```python
from build123d import *

# Parameters (mm, degrees)
SKETCH_1_W             = 230.160423268
SKETCH_1_H             = 76.880643476
SM_BASE_FLANGE_1_DEPTH = 1
OTHER_START            = -38.440321738
OTHER_1_DEPTH          = 76.880643476
OTHER_1_2_DEPTH        = 76.880643476


# Read off the part's stored shape, not the designer's step: 转折1
# Sheet-metal steps are written as plain solids
with BuildPart() as part:
    # Sketch 1 → 基体-法兰1 (new body)
    with BuildSketch(Plane(origin=(0, 0, 0), x_dir=(1, 0, 0), z_dir=(0, 1, 0))):
        Rectangle(SKETCH_1_W, SKETCH_1_H)
    extrude(amount=-SM_BASE_FLANGE_1_DEPTH)

    # Other 1 outline → Other 1 (cut)
    with BuildSketch(Plane.XY.offset(OTHER_START)):
        with BuildLine():
            Line((115.080211634, 0), (0.093295252, 0))
            ThreePointArc((0.093295252, 0), (-1.033318835, -0.740370349), (-2.35619449, -1))
            Line((-2.35619449, -1), (115.080211634, -1))
            Line((115.080211634, -1), (115.080211634, 0))
        make_face()
    extrude(amount=OTHER_1_DEPTH, mode=Mode.SUBTRACT)

    # Other 1 2 outline → Other 1 2 (add)
    with BuildSketch(Plane.XY.offset(OTHER_START)):
        with BuildLine():
            ThreePointArc((3.64380551, 51), (1.168931776, 49.974873734), (0.14380551, 47.5))
            Line((0.14380551, 47.5), (0.14380551, 2.5))
            ThreePointArc((0.14380551, 2.5), (-0.588427537, 0.732233047), (-2.35619449, 0))
            Line((-2.35619449, 0), (0.093295252, 0))
            ThreePointArc((0.093295252, 0), (0.870507704, 1.144126499), (1.14380551, 2.5))
            Line((1.14380551, 2.5), (1.14380551, 47.5))
            ThreePointArc((1.14380551, 47.5), (1.876038557, 49.267766953), (3.64380551, 50))
            Line((3.64380551, 50), (115.080211634, 50))
            Line((115.080211634, 50), (115.080211634, 51))
            Line((115.080211634, 51), (3.64380551, 51))
        make_face()
    extrude(amount=OTHER_1_2_DEPTH)


solid = part.part
```
For this review, take the finished solid that the model builds, in its own axes (mm). A direction names the side the tool comes from. Coordinates: 2 decimals unless noted, no trailing zeros. Loops run counter-clockwise (first coordinate to the right, second up) from the corner with the lowest first, then second, coordinate; pieces in that order, holes last. Notation, with made-up numbers: (-38.5, 0) - (-0.5, 0) arc R18 ccw to (-0.5, 6) - close; hole circle Ø9 at (18, 26). An arc over 180 degrees is marked (long way). Use one line per item in the form item = value. Start each with the question number.
1) To check wall thickness, follow probe 1 along Y at (x, z) = (63, 19); probe 2 along Y at (x, z) = (-91, -7); probe 3 along X at (y, z) = (9.5, -18.5). State the ranges of each line that lie inside material, in increasing order. Write a range as from..to.
2) Take a section at C-C (y = 22). State the section outline as (x, z) points.
3) Take a section at A-A (z = -7). State the section outline as (x, y) points.
4) For faces 1 (the face through (0.144, 25, -1)), 2 (the face through (1.144, 25, -1)), 3 (the face through (50.6, 50.2, -38.44)), list the 3-axis set-ups (+Z, -Z, +X, -X, +Y, -Y) from which the entire face can be reached by the end or side of a thin tool; tool diameter is ignored.
5) For pin 1 (1 mm diameter, centred on x = 34, z = 9.5, fed in from -Y); pin 2 (2 mm diameter, centred on y = 28, z = -6.5, fed in from -X); pin 3 (3 mm diameter, centred on x = -31, z = 8.5, fed in from +Y), all flat-tipped, find the tip position at first contact; note any pin that passes through.
6) Take a section at B-B (x = 24). State the section outline as (y, z) points, plus the area to 3 significant figures.
From the geometry:
q1.probe_1 = 50..51
q1.probe_2 = -1..0
q1.probe_3 = 0.14..1.14
q2.outline = (0.14, -38.44) - (1.14, -38.44) - (1.14, 38.44) - (0.14, 38.44) - close
q3.outline = (-115.08, -1) - (-2.36, -1) arc R3.5 ccw to (1.14, 2.5) - (1.14, 47.5) arc R2.5 cw to (3.64, 50) - (115.08, 50) - (115.08, 51) - (3.64, 51) arc R3.5 ccw to (0.14, 47.5) - (0.14, 2.5) arc R2.5 cw to (-2.36, 0) - (-115.08, 0) - close
q4.face_1 = +Z, -Z, -X, +Y
q4.face_2 = +Z, -Z, +X, -Y
q4.face_3 = -Z, +X, -X, +Y, -Y
q5.pin_1 = 50
q5.pin_2 = 0.14
q5.pin_3 = 0
q6.outline = (50, -38.44) - (51, -38.44) - (51, 38.44) - (50, 38.44) - close
q6.area = 76.9 mm2
